Check sheet for the modelled part. Datum: model origin and axes. Units: mm. Round coordinates to 2 decimals unless told otherwise and drop trailing zeros. Write each loop counter-clockwise with the first axis right and the second up, starting at its lowest first coordinate (ties: lowest second). Pieces come first, ordered by that corner, then holes. Notation, with made-up numbers: (25.5, 62) - (43.5, 62) arc R24 ccw to (43.5, 90) - close; hole circle Ø9 at (54.25, 3). An arc over 180 degrees is marked (long way). Answer as a JSON object with one key per item and string values. Group by question number.
Item 1: Sectioned sample at B-B on z = 0.65. Record the boundary of the cut face in (x, y).
Item 2: Sectioned sample at A-A on x = 232. Record the boundary of the cut face in (y, z), plus the area to 3 significant figures.
Item 3: Sectioned sample at C-C on x = 164. Record the boundary of the cut face in (y, z).
Item 4: Release check for a two-part mould opening along Y. For faces 1 (the cylindrical face through (241.496, 0.288, 0.592)), 2 (the flat face through (1, 1, 1.2)), 3 (the cylindrical face through (-236.046, 0.178, 0.592)) record: pulls with the +Y half, pulls with the -Y half, needs draft (parallel to the pull), parting line crosses it, or undercut.
Item 5: Thickness scan on line 1 (Y direction, x = -232, z = 0.6); line 2 (Y direction, x = -49, z = 0.35); line 3 (X direction, y = -2.25, z = 0.3). Record the ranges inside material, lowest first.
Item 6: Gauge pin test, flat ends, axial feed: P1, Ø10.5, axis at x = -232, y = 0, coming from the -Z side; P2, Ø0.6, axis at x = -63, z = 0.5, coming from the -Y side. Record the tip position at first contact, or that the pin passes through.
```python
from build123d import *

# Parameters (mm, degrees)
SKETCH1_R           = 4.05
BOSS_EXTRUDE1_DEPTH = 1.2


with BuildPart() as part:
    # Sketch1 → Boss-Extrude1 (new body)
    with BuildSketch(Plane.XY):
        with BuildLine():
            Line((2.50049995, 3.5), (212.557777905, 3.5))
            ThreePointArc((212.557777905, 3.5), (219.929875713, 4.611672852), (226.64634464, 7.847826087))
            ThreePointArc((226.64634464, 7.847826087), (241.5, 0), (226.64634464, -7.847826087))
            ThreePointArc((226.64634464, -7.847826087), (219.929875713, -4.611672852), (212.557777905, -3.5))
            Line((212.557777905, -3.5), (2.50049995, -3.5))
            ThreePointArc((2.50049995, -3.5), (2.183498063, -3.386664976), (2.010205842, -3.098039216))
            ThreePointArc((2.010205842, -3.098039216), (0, -1.45), (-2.010205842, -3.098039216))
            ThreePointArc((-2.010205842, -3.098039216), (-2.183498063, -3.386664976), (-2.50049995, -3.5))
            Line((-2.50049995, -3.5), (-212.557777905, -3.5))
            ThreePointArc((-212.557777905, -3.5), (-219.929875713, -4.611672852), (-226.64634464, -7.847826087))
            ThreePointArc((-226.64634464, -7.847826087), (-241.5, 0), (-226.64634464, 7.847826087))
            ThreePointArc((-226.64634464, 7.847826087), (-219.929875713, 4.611672852), (-212.557777905, 3.5))
            Line((-212.557777905, 3.5), (-2.50049995, 3.5))
            ThreePointArc((-2.50049995, 3.5), (-2.183498063, 3.386664976), (-2.010205842, 3.098039216))
            ThreePointArc((-2.010205842, 3.098039216), (0, 1.45), (2.010205842, 3.098039216))
            ThreePointArc((2.010205842, 3.098039216), (2.183498063, 3.386664976), (2.50049995, 3.5))
        make_face()
        with Locations((232, 0)):
            Circle(SKETCH1_R, mode=Mode.SUBTRACT)
        with Locations((-232, 0)):
            Circle(SKETCH1_R, mode=Mode.SUBTRACT)
    extrude(amount=BOSS_EXTRUDE1_DEPTH)


solid = part.part
```
Completed:
{
 "1": {"outline": "(-226.65, -7.85) arc R25 cw to (-212.56, -3.5) - (-2.5, -3.5) arc R0.5 ccw to (-2.01, -3.1) arc R2.05 cw to (2.01, -3.1) arc R0.5 ccw to (2.5, -3.5) - (212.56, -3.5) arc R25 cw to (226.65, -7.85) arc R9.5 ccw (long way) to (226.65, 7.85) arc R25 cw to (212.56, 3.5) - (2.5, 3.5) arc R0.5 ccw to (2.01, 3.1) arc R2.05 cw to (-2.01, 3.1) arc R0.5 ccw to (-2.5, 3.5) - (-212.56, 3.5) arc R25 cw to (-226.65, 7.85) arc R9.5 ccw (long way) to start; hole circle Ø8.1 at (-232, 0); hole circle Ø8.1 at (232, 0)"},
 "2": {"outline": "(-9.5, 0) - (-4.05, 0) - (-4.05, 1.2) - (-9.5, 1.2) - close; (4.05, 0) - (9.5, 0) - (9.5, 1.2) - (4.05, 1.2) - close", "area": "13.1 mm²"},
 "3": {"outline": "(-3.5, 0) - (3.5, 0) - (3.5, 1.2) - (-3.5, 1.2) - close"},
 "4": {"face 1": "parting line crosses it", "face 2": "needs draft", "face 3": "undercut"},
 "5": {"line 1": "-9.5 to -4.05, 4.05 to 9.5", "line 2": "-3.5 to 3.5", "line 3": "-241.23 to -235.37, -228.63 to -1.62, 1.62 to 228.63, 235.37 to 241.23"},
 "6": {"P1": "z = 0", "P2": "y = -3.5"}
}
